Could you check a few things on this drawing? It's one solid part, dimensions in mm from its lowest x, y, z. Coordinates: 2 decimals unless noted, no trailing zeros. Order: outer loops, then holes, each group sorted by start corner. A loop starts at its lowest first (then second) coordinate and runs counter-clockwise, first axis right, second up. Notation, with made-up numbers: (75, -6.5) - (90, -6.5) arc R34 cw to (90, 24.5) - close; hole circle Ø3 at (64, 46.25). An arc over 180 degrees is marked (long way). Answer in a Markdown table with one row per item. Add a question column.
Item 1: I want a section at A-A (x = 10.35). Please give me the cut outline in (y, z).
Item 2: Will this pin go through, and if not, where does the flat tip stop? pin 1 Ø3 at (x, y) = (5.08, 5.08) entering from +Z.
Item 3: I want a section at B-B (y = 48.85). Please give me the cut outline in (x, z).
Item 4: I want a section at C-C (z = 1.35). Count the separate pieces of the cut face and the enclosed holes in it, plus the area to 3 significant figures.
Item 5: If I drill on line 1 along Y through (x, z) = (37.35, 0.55); line 2 along Y through (x, z) = (38.5, 0.4); line 3 along X through (y, z) = (71.12, 0.95) (3 decimals), over which ranges is the centre line in solid material (lowest first)? Write a range as from..to.
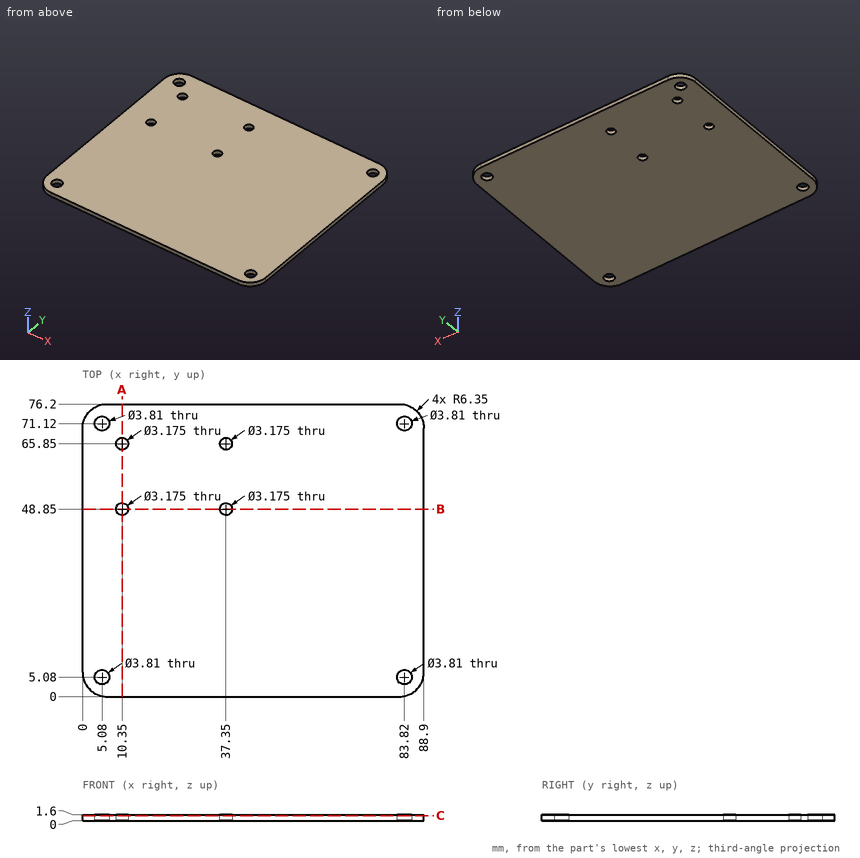
Values follow:
| question | item | result |
|---|---|---|
| 1 | outline | (0, 0) - (47.26, 0) - (47.26, 1.6) - (0, 1.6) - close; (50.44, 0) - (64.26, 0) - (64.26, 1.6) - (50.44, 1.6) - close; (67.44, 0) - (76.2, 0) - (76.2, 1.6) - (67.44, 1.6) - close |
| 2 | pin 1 | passes through |
| 3 | outline | (0, 0) - (8.76, 0) - (8.76, 1.6) - (0, 1.6) - close; (11.94, 0) - (35.76, 0) - (35.76, 1.6) - (11.94, 1.6) - close; (38.94, 0) - (88.9, 0) - (88.9, 1.6) - (38.94, 1.6) - close |
| 4 | separate pieces | 1 |
| 4 | enclosed holes | 8 |
| 4 | area | 6,660 mm^2 |
| 5 | line 1 | y = 0..47.26, 50.44..64.26, 67.44..76.2 |
| 5 | line 2 | y = 0..47.76, 49.94..64.76, 66.94..76.2 |
| 5 | line 3 | x = 0.128..3.175, 6.985..81.915, 85.725..88.772 |
